from build123d import *

# Parameters (mm, degrees)
F1_DEPTH = 25.4


with BuildPart() as f1:
    # F0 (on Front) → F1 (new body)
    with BuildSketch(Plane.XZ):
        Polygon((-11.412839, 43.004113), (-47.613019, -34.627423), (-25.406242, -34.627423), (-9.081334, 0.381454), (18.921843, 0.381454), (36.686134, -32.201932), (58.23868, -32.201932), (17.236739, 43.004113), align=None)
        Polygon((-7.921455, 17.322859), (-3.90137, 28.367954), (8.457227, 28.367954), (12.477313, 17.322859), align=None, mode=Mode.SUBTRACT)
    extrude(amount=F1_DEPTH)


solid = f1.part
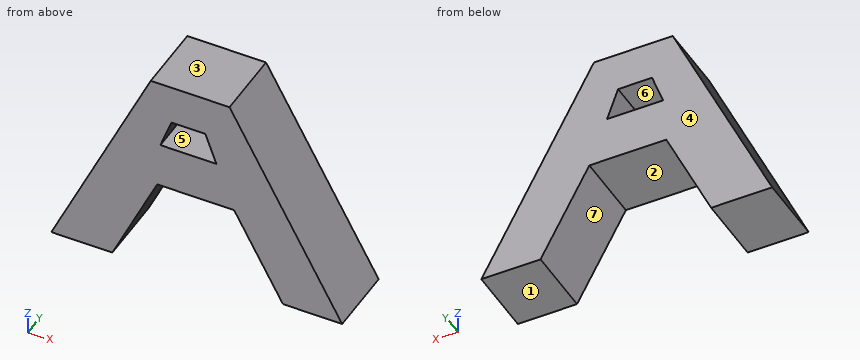
The listing builds one solid part. Answer for the finished solid, in the listing's coordinates (mm). Face numbers are marked on the shaded views. A direction names the side the tool comes from. Give positions to 0.01 mm unless a question says otherwise; leave off trailing zeros. Write each loop counter-clockwise with the first axis right and the second up, starting at its lowest first coordinate (ties: lowest second). Pieces come first, ordered by that corner, then holes.
Item 1: Section D-D, the plane x = -26.5 is taken. Write down the section's boundary in (y, z).
Item 2: Section B-B, the plane y = -18 is taken. Write down the section's boundary in (x, z), plus the area to 3 significant figures.
Item 3: Which of the six approach directions +Z, -Z, +X, -X, +Y, -Y give full straight-line access (tool end or side, diameter ignored) to the marked faces 1, 2 and 3?
Item 4: Flat-ended cylindrical pins translate along their axes: P1, Ø3, axis at y = -21, z = -22.5, coming from the +X side; P2, Ø12, axis at x = -2, y = -4.5, coming from the -Z side; P3, Ø2, axis at y = -21, z = -5, coming from the -X side. Find the tip coordinate at first contact, or state that the pin passes through.
Item 5: Section C-C, the plane z = 25 is taken. Write down the section's boundary in (x, y), plus the area to 3 significant figures.
Item 6: Section A-A, the plane x = 7 is taken. Write down the section's boundary in (y, z).
Item 7: Find the intervals of material crossed by line 1 along Z through (x, y) = (6, -17.25); line 2 along X through (y, z) = (-5, -13.5); line 3 along X through (y, z) = (-9.25, -19), in increasing order.
Item 8: Determine the mould class of the marked faces 4, 5, 6 and 7 for opening direction Z: released by +Z, released by -Z, zero draft, split by the parting line, or undercut.
Completed:
1. outline: (-25.4, -34.63) - (0, -34.63) - (0, 10.65) - (-25.4, 10.65) - close
2. outline: (-47.61, -34.63) - (-25.41, -34.63) - (-9.08, 0.38) - (18.92, 0.38) - (36.69, -32.2) - (58.24, -32.2) - (17.24, 43) - (-11.41, 43) - close; hole (-7.92, 17.32) - (12.48, 17.32) - (8.46, 28.37) - (-3.9, 28.37) - close
2. area: 3,440 mm2
3. face 1: -Z, +X, +Y, -Y
3. face 2: -Z, +Y, -Y
3. face 3: +Z, +X, -X, +Y, -Y
4. P1: stops at x = 53.77
4. P2: stops at z = 0.38
4. P3: stops at x = -34.26
5. outline: (-19.81, -25.4) - (-5.13, -25.4) - (-5.13, 0) - (-19.81, 0) - close; (9.68, -25.4) - (27.05, -25.4) - (27.05, 0) - (9.68, 0) - close
5. area: 814 mm2
6. outline: (-25.4, 0.38) - (0, 0.38) - (0, 17.32) - (-25.4, 17.32) - close; (-25.4, 28.37) - (0, 28.37) - (0, 43) - (-25.4, 43) - close
7. line 1: z = 0.38 to 17.32, 28.37 to 43
7. line 2: x = -37.76 to -15.55, 26.49 to 48.04
7. line 3: x = -40.33 to -18.12, 29.49 to 51.04
8. face 4: zero draft
8. face 5: undercut
8. face 6: undercut
8. face 7: released by -Z
